```python
from build123d import *

# Parameters (mm, degrees)
F0_W     = 19.05
F0_H     = 31.75
F1_DEPTH = 31.75
F2_T     = -2.54
F4_R     = 4.6736
F4_R_2   = 3.5941
F5_DEPTH = 5.08
F6_R     = 1.27


# Not quite as in the source:
# - a feature names something its author has since deleted; it is built from what else it names


with BuildPart() as f1:
    # F0 (on Top) → F1 (new body)
    with BuildSketch(Plane.XY):
        with Locations((-14.8217186228, -11.3360365331)):
            Rectangle(F0_W, F0_H)
    extrude(amount=F1_DEPTH)

    # F2
    f2_openings = [f1.faces().sort_by_distance(p)[0] for p in [
        (-5.296719, -11.336037, 15.875),
    ]]
    offset(amount=F2_T, openings=f2_openings)

    # F4 (on face) → F5 (join)
    with BuildSketch(Plane(origin=(-24.3467186228, 0, 0), x_dir=(0, -1, 0), z_dir=(-1, 0, 0))):
        with Locations((19.3370365331, 23.876)):
            Circle(F4_R)
        with Locations((19.3370365331, 23.876)):
            Circle(F4_R_2, mode=Mode.SUBTRACT)
        with Locations((3.2080365331, 23.876)):
            Circle(F4_R)
        with Locations((3.2080365331, 23.876)):
            Circle(F4_R_2, mode=Mode.SUBTRACT)
        with Locations((3.3106288512, 7.8743288743)):
            Circle(F4_R)
        with Locations((3.3106288512, 7.8743288743)):
            Circle(F4_R_2, mode=Mode.SUBTRACT)
        with Locations((19.4396288512, 7.8743288743)):
            Circle(F4_R)
        with Locations((19.4396288512, 7.8743288743)):
            Circle(F4_R_2, mode=Mode.SUBTRACT)
    extrude(amount=F5_DEPTH)

    # F6
    f6_edges = [f1.edges().sort_by_distance(p)[0] for p in [
        (-14.821719, 4.538963, 0),
        (-24.346719, -11.336037, 0),
        (-14.821719, -27.211037, 0),
        (-5.296719, -11.336037, 0),
        (-24.346719, -27.211037, 15.875),
        (-14.821719, 4.538963, 31.75),
        (-24.346719, -11.336037, 31.75),
        (-14.821719, -27.211037, 31.75),
        (-5.296719, -11.336037, 31.75),
        (-5.296719, -27.211037, 15.875),
        (-5.296719, 4.538963, 15.875),
        (-24.346719, 4.538963, 15.875),
    ]]
    fillet(f6_edges, radius=F6_R)


solid = f1.part
```
CAD build for the part. Positions are in the model's coordinates, mm. A direction names the side the tool comes from. Round coordinates to 2 decimals unless told otherwise and drop trailing zeros. Write each loop counter-clockwise with the first axis right and the second up, starting at its lowest first coordinate (ties: lowest second). Pieces come first, ordered by that corner, then holes. Notation, with made-up numbers: (-22.75, -35) - (22.25, -35) arc R18 cw to (22.25, -27) - close; hole circle Ø11 at (59.5, 16.5). An arc over 180 degrees is marked (long way). Write item = value, one per line. Start each with the question number.
Q1. Band-saw the part on A-A (x = -7.25). Give the cut face in (y, z).
Q2. Band-saw the part on B-B (y = -8.5). Give the cut face in (x, z), then the cut area to 3 significant figures.
Q3. Drop flat-ended pins along their axis: pin 1 (3.5 mm diameter, centred on y = -19, z = 24, fed in from -X); pin 2 (4.5 mm diameter, centred on y = -19.34, z = 23.88, fed in from +X). Give the stop position or say it passes through.
Q4. Which spindle directions (+Z, -Z, +X, -X, +Y, -Y) get a long thin tool onto all of the face, cutting with end or side? Do faces 1 (the cylindrical face through (-26.85, -15.99, 11.03)), 2 (the flat face through (-15, -11, 31.75)), 3 (the flat face through (-14, -24.671, 16)). Say none if no direction does.
Q5. Band-saw the part on C-C (x = -25.75). Give the cut face in (y, z).
Q6. Band-saw the part on D-D (z = 18.5). Give the cut face in (x, y).
Q7. Probe L1, parallel to Z at x = -12.5, y = -2.5; L2, parallel to Y at x = -14, z = 24.5; L3, parallel to Z at x = -26.75, y = -6. List the from-to ranges inside material, lowest first. Write a range as from..to.
Q8. Mould opens along Y. For faces 4 (the flat face through (-21.807, -12, 16)), 5 (the flat face through (-5.297, -12, 30)), 6 (the flat face through (-14, -11, 2.54)), 7 (the flat face through (-15, 4.539, 16)) say: pulls with the +Y half, pulls with the -Y half, needs draft (parallel to the pull), parting line crosses it, or undercut.
Answers below:
q1.outline = (-27.21, 1.27) arc R1.27 ccw to (-25.94, 0) - (3.27, 0) arc R1.27 ccw to (4.54, 1.27) - (4.54, 30.48) arc R1.27 ccw to (3.27, 31.75) - (-25.94, 31.75) arc R1.27 ccw to (-27.21, 30.48) - close; hole (-24.67, 2.54) - (2, 2.54) - (2, 29.21) - (-24.67, 29.21) - close
q2.outline = (-24.35, 1.27) arc R1.27 ccw to (-23.08, 0) - (-6.57, 0) arc R1.27 ccw to (-5.3, 1.27) - (-5.3, 2.54) - (-21.81, 2.54) - (-21.81, 29.21) - (-5.3, 29.21) - (-5.3, 30.48) arc R1.27 ccw to (-6.57, 31.75) - (-23.08, 31.75) arc R1.27 ccw to (-24.35, 30.48) - close
q2.area = 163 mm2
q3.pin_1 = -24.35
q3.pin_2 = -21.81
q4.face_1 = -X
q4.face_2 = +Z, +X, -X, +Y, -Y
q4.face_3 = +X
q5.outline = circle Ø9.35 at (-19.44, 7.87); circle Ø9.35 at (-19.34, 23.88); circle Ø9.35 at (-3.31, 7.87); circle Ø9.35 at (-3.21, 23.88); hole circle Ø7.19 at (-19.44, 7.87); hole circle Ø7.19 at (-19.34, 23.88); hole circle Ø7.19 at (-3.31, 7.87); hole circle Ø7.19 at (-3.21, 23.88)
q6.outline = (-24.35, -25.94) arc R1.27 ccw to (-23.08, -27.21) - (-6.57, -27.21) arc R1.27 ccw to (-5.3, -25.94) - (-5.3, -24.67) - (-21.81, -24.67) - (-21.81, 2) - (-5.3, 2) - (-5.3, 3.27) arc R1.27 ccw to (-6.57, 4.54) - (-23.08, 4.54) arc R1.27 ccw to (-24.35, 3.27) - close
q7.L1 = 0..2.54, 29.21..31.75
q7.L2 = -27.21..-24.67, 2..4.54
q7.L3 = 4.05..5.49, 10.26..11.7, 20.13..21.61, 26.14..27.62
q8.face_4 = undercut
q8.face_5 = needs draft
q8.face_6 = undercut
q8.face_7 = pulls with the +Y half
